from build123d import *

# Parameters (mm, degrees)
F0_R          = 2.5
F1_DEPTH      = 15
F1_DEPTH_BACK = 15
F2_DEPTH      = 12.5
F2_DEPTH_BACK = 12.5
F4_DEPTH      = 5
F6_DEPTH      = 40.001


with BuildPart() as f1:
    # F0 (on Right) → F1 (new body, two sides)
    with BuildSketch(Plane.YZ) as f1_sk:
        with BuildLine():
            ThreePointArc((97.5, -10), (104.571068, -7.071068), (107.5, 0))
            ThreePointArc((107.5, 0), (104.571068, 7.071068), (97.5, 10))
            Line((97.5, 10), (96.526706, 9.952522))
            ThreePointArc((96.526706, 9.952522), (87.511876, -0.487226), (97.5, -10))
        make_face()
        with Locations((97.5, 0)):
            Circle(F0_R, mode=Mode.SUBTRACT)
    extrude(amount=F1_DEPTH)
    extrude(f1_sk.sketch, amount=-F1_DEPTH_BACK)

    # F0 (on Right) → F2 (join, two sides)
    with BuildSketch(Plane.YZ) as f2_sk:
        with BuildLine():
            Line((-107.5, -10), (97.5, -10))
            ThreePointArc((97.5, -10), (87.511876, -0.487226), (96.526706, 9.952522))
            Line((96.526706, 9.952522), (-107.5, 0))
            Line((-107.5, 0), (-107.5, -10))
        make_face()
    extrude(amount=F2_DEPTH)
    extrude(f2_sk.sketch, amount=-F2_DEPTH_BACK)

    # F3 (on face) → F4 (cut)
    with BuildSketch(Plane(origin=(0, 0, -10), x_dir=(1, 0, 0), z_dir=(0, 0, -1))):
        Polygon((9, -67.5), (9, 105), (-9, 105), (-9, -67.5), (0, -67.5), align=None)
    extrude(amount=-F4_DEPTH, mode=Mode.SUBTRACT)

    # F5 (on face) → F6 (cut, through all)
    with BuildSketch(Plane.XZ.offset(-67.5)):
        Polygon((-1, -10), (0, -10), (1, -10), (1, -5), (0, -5), (-1, -5), align=None)
    extrude(amount=-F6_DEPTH, mode=Mode.SUBTRACT)


solid = f1.part
Check sheet for the modelled part. Datum: model origin and axes. Units: mm. A direction names the side the tool comes from. Give positions to 0.01 mm unless a question says otherwise; leave off trailing zeros. Loops run counter-clockwise (first coordinate to the right, second up) from the corner with the lowest first, then second, coordinate; pieces in that order, holes last. Notation, with made-up numbers: M 73,19.25 L 93,19.25 A16 cw 93,41.25 Z; hole C 7.5,48 d2. An arc over 180 degrees is marked long. Answer as a JSON object with one key per item and string values. Group by question number.
Q1. Cross-section at A-A on x = 6.25. Record the cut outline in (y, z).
Q2. Material ranges on line 1 along X through (y, z) = (29, -5.75); line 2 along Z through (x, y) = (-9, 97.5); line 3 along X through (y, z) = (-50.5, 2.75), recorded low to high. Write a range as [from, to].
Q3. Cross-section at C-C on z = -7.75. Record the cut outline in (x, y), then the cut area to 3 significant figures.
Q4. Cross-section at B-B on y = 6. Record the cut outline in (x, z), then the cut area to 3 significant figures.
Q5. Access from +Z, -Z, +X, -X, +Y, -Y to the whole of each face (thin tool, end or side, straight path). Record for faces 4 (the flat face through (-1, 87, -7)), 5 (the flat face through (9, -18, -8)), 6 (the flat face through (0, -107.5, -5)).
Q6. Release check for a two-part mould opening along X. For faces 1 (the flat face through (1, 87, -8)), 2 (the cylindrical face through (0, 96, -2)), 3 (the flat face through (-15, 100, -2)) record: released by +X, released by -X, zero draft, split by the parting line, or undercut.
Q7. Go/stop test with flat-tipped pins: P1, Ø4, axis at x = -1.5, z = -7.5, coming from the +Y side; P2, Ø4, axis at y = 78, z = -6.5, coming from the -X side; P3, Ø4, axis at y = 79.5, z = -6.5, coming from the +X side; P4, Ø12, axis at x = -9, z = 5, coming from the -Y side. Record where each tip stops, or that it passes through.
Q8. Cross-section at D-D on y = -70.5. Record the cut outline in (x, z), then the cut area to 3 significant figures.
Evaluation:
{
 "1": {"outline": "M -107.5,-10 L -105,-10 L -105,-5 L 67.5,-5 L 67.5,-10 L 97.5,-10 A10 ccw 107.5,0 A10 ccw 97.5,10 L 96.53,9.95 L -107.5,0 Z; hole C 97.5,0 d5"},
 "2": {"line 1": "x = [-12.5, -9], [9, 12.5]", "line 2": "z = [-10, -2.5], [2.5, 10]", "line 3": "x = [-12.5, 12.5]"},
 "3": {"outline": "M -15,91.18 L -12.5,91.18 L -12.5,-107.5 L 12.5,-107.5 L 12.5,91.18 L 15,91.18 L 15,103.82 L 1,103.82 L 1,67.5 L 9,67.5 L 9,-105 L -9,-105 L -9,67.5 L -1,67.5 L -1,103.82 L -15,103.82 Z", "area": "2,170 mm2"},
 "4": {"outline": "M -12.5,-10 L -9,-10 L -9,-5 L 9,-5 L 9,-10 L 12.5,-10 L 12.5,5.54 L -12.5,5.54 Z", "area": "298 mm2"},
 "5": {"face 4": "-Z, +Y", "face 5": "-Z", "face 6": "+Z, -Z, +X, -X, -Y"},
 "6": {"face 1": "undercut", "face 2": "zero draft", "face 3": "released by -X"},
 "7": {"P1": "stops at y = 105.85", "P2": "stops at x = -12.5", "P3": "stops at x = 12.5", "P4": "stops at y = -107.5"},
 "8": {"outline": "M -12.5,-10 L -9,-10 L -9,-5 L 9,-5 L 9,-10 L 12.5,-10 L 12.5,1.8 L -12.5,1.8 Z", "area": "205 mm2"}
}
